Here's the drawing with two shaded views (mm, measured from the low corner). I have some questions. Give positions to 0.01 mm unless a question says otherwise; leave off trailing zeros. Order: outer loops, then holes, each group sorted by start corner. A loop starts at its lowest first (then second) coordinate and runs counter-clockwise, first axis right, second up. Notation, with made-up numbers: M 12.5,14.5 L 40.5,14.5 A21 cw 40.5,37.5 Z; hole C 54,-35.75 d5. An arc over 180 degrees is marked long. Use a Markdown table: item, result. Add a question column.
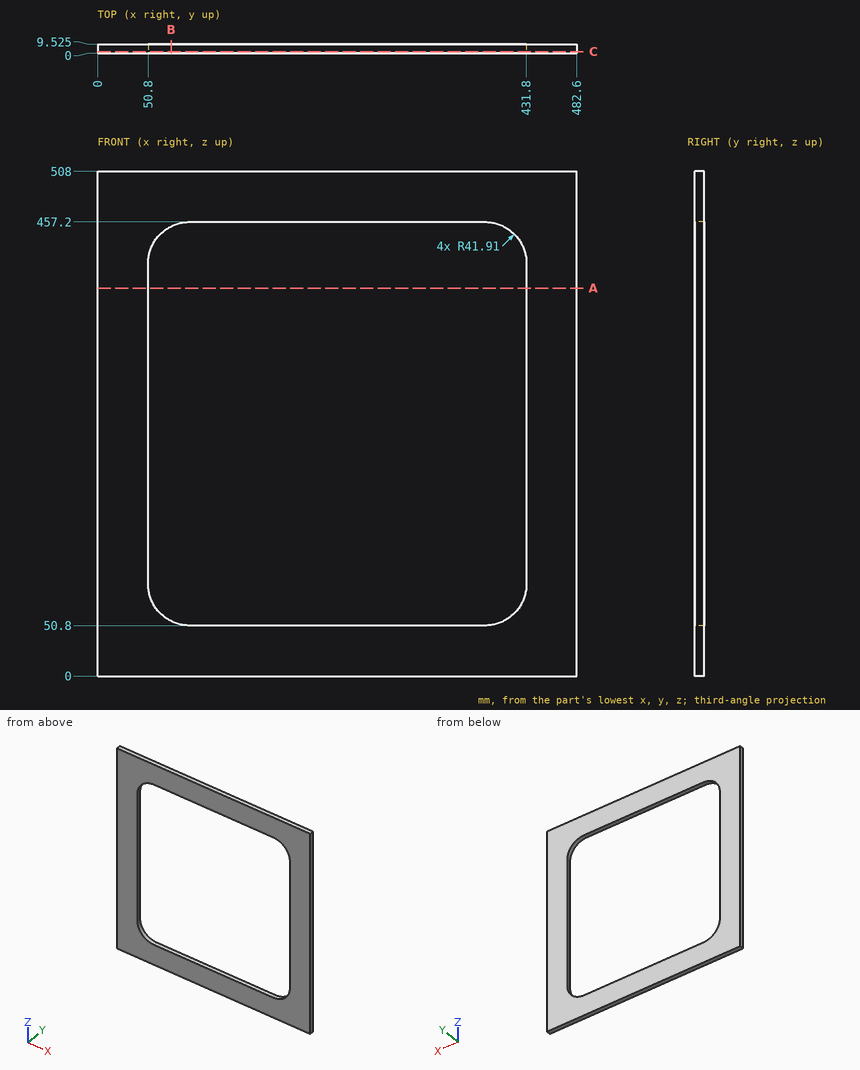
1. If we section it at C-C, the plane y = 1.75: List the corners of the cut face in (x, z) for me, then the cut area to 3 significant figures.
2. I need wall thicknesses on L1, parallel to X at y = 9, z = 325; L2, parallel to Z at x = 316.5, y = 2; L3, parallel to X at y = 0.5, z = 63. Which ranges of each line are inside material? Lowest first, please. Write a range as [from, to].
3. If we section it at B-B, the plane x = 74: List the corners of the cut face in (y, z) for me (3 decimals), then the cut area to 3 significant figures.
4. If we section it at A-A, the plane z = 390.5: List the corners of the cut face in (x, y) for me (3 decimals), then the cut area to 3 significant figures.
Geometry results:
| question | item | result |
|---|---|---|
| 1 | outline | M 0,0 L 482.6,0 L 482.6,508 L 0,508 Z; hole M 50.8,92.71 A41.91 ccw 92.71,50.8 L 389.89,50.8 A41.91 ccw 431.8,92.71 L 431.8,415.29 A41.91 ccw 389.89,457.2 L 92.71,457.2 A41.91 ccw 50.8,415.29 Z |
| 1 | area | 91,800 mm^2 |
| 2 | L1 | x = [0, 50.8], [431.8, 482.6] |
| 2 | L2 | z = [0, 50.8], [457.2, 508] |
| 2 | L3 | x = [0, 63.15], [419.45, 482.6] |
| 3 | outline | M 0,0 L 9.525,0 L 9.525,55.208 L 0,55.208 Z; M 0,452.792 L 9.525,452.792 L 9.525,508 L 0,508 Z |
| 3 | area | 1,050 mm^2 |
| 4 | outline | M 0,0 L 50.8,0 L 50.8,9.525 L 0,9.525 Z; M 431.8,0 L 482.6,0 L 482.6,9.525 L 431.8,9.525 Z |
| 4 | area | 968 mm^2 |
